Source: CAD feature listing. Evaluate the final solid. Frame: model axes, mm. A direction names the side the tool comes from. Coordinates: 2 decimals unless noted, no trailing zeros. Loops run counter-clockwise (first coordinate to the right, second up) from the corner with the lowest first, then second, coordinate; pieces in that order, holes last.
Item 1: Section query A-A, the plane y = 84.5. Return the cut outline in (x, z).
Item 2: Pull-direction query (X, two-part tool) for faces 3 (the flat face through (80, 59, 26)), 4 (the flat face through (78.5, 61, 26)), 5 (the flat face through (74, 121.5, 26)); classes: +X half, -X half, draft (parallel to the pull), parting line (faces both ways), or undercut.
Item 3: Section query B-B, the plane x = 7. Return the cut outline in (y, z), then the cut area to 3 significant figures.
Item 4: Reachability of faces 1 (the flat face through (-74, 121.5, 26)), 2 (the flat face through (1, 0, 20)) from +Z, -Z, +X, -X, +Y, -Y: full face, straight path, thin tool, end or side. Return the list, or none.
Item 5: Pin query (flat end, axial travel): pin 1 Ø1.2 at (y, z) = (-1, 45) entering from -X; pin 2 Ø1.2 at (y, z) = (-1, 45.5) entering from +X; pin 3 Ø1.6 at (y, z) = (120.5, 38.5) entering from +X. Return the tip coordinate at first contact, or that it passes through.
Item 6: Section query C-C, the plane z = 32.5. Return the cut outline in (x, y).
Item 7: Line query: probe 1 along X at (y, z) = (40, 35.5); probe 2 along Y at (x, z) = (-66, 12). Output: solid intervals per line, ascending.
```python
from build123d import *

# Parameters (mm, degrees)
F1_DEPTH = 52
F3_DEPTH = 123.001


with BuildPart() as f1:
    # F0 (on Top) → F1 (new body)
    with BuildSketch(Plane.XY):
        with BuildLine():
            Line((78, 0), (0, 0))
            Line((0, 0), (-78, 0))
            ThreePointArc((-78, 0), (-78.353553, 0.146447), (-78.5, 0.5))
            Line((-78.5, 0.5), (-78.5, 119.5))
            ThreePointArc((-78.5, 119.5), (-78.353553, 119.853553), (-78, 120))
            Line((-78, 120), (-70, 120))
            Line((-70, 120), (-70, 121.5))
            Line((-70, 121.5), (-78, 121.5))
            ThreePointArc((-78, 121.5), (-79.414214, 120.914214), (-80, 119.5))
            Line((-80, 119.5), (-80, 0.5))
            ThreePointArc((-80, 0.5), (-79.414214, -0.914214), (-78, -1.5))
            Line((-78, -1.5), (0, -1.5))
            Line((0, -1.5), (78, -1.5))
            ThreePointArc((78, -1.5), (79.414214, -0.914214), (80, 0.5))
            Line((80, 0.5), (80, 119.5))
            ThreePointArc((80, 119.5), (79.414214, 120.914214), (78, 121.5))
            Line((78, 121.5), (70, 121.5))
            Line((70, 121.5), (70, 120))
            Line((70, 120), (78, 120))
            ThreePointArc((78, 120), (78.353553, 119.853553), (78.5, 119.5))
            Line((78.5, 119.5), (78.5, 0.5))
            ThreePointArc((78.5, 0.5), (78.353553, 0.146447), (78, 0))
        make_face()
    extrude(amount=F1_DEPTH)

    # F2 (on face) → F3 (cut, through all)
    with BuildSketch(Plane.XZ.offset(1.5)):
        Polygon((0, 50), (-70, 50), (-70, 42), (0, 42), (70, 42), (70, 50), align=None)
    extrude(amount=-F3_DEPTH, mode=Mode.SUBTRACT)


solid = f1.part
```
Verdict:
1. outline: (-80, 0) - (-78.5, 0) - (-78.5, 52) - (-80, 52) - close; (78.5, 0) - (80, 0) - (80, 52) - (78.5, 52) - close
2. face 3: +X half
2. face 4: undercut
2. face 5: draft
3. outline: (-1.5, 0) - (0, 0) - (0, 42) - (-1.5, 42) - close; (-1.5, 50) - (0, 50) - (0, 52) - (-1.5, 52) - close
3. area: 66.0 mm2
4. face 1: +Z, -Z, +X, -X, +Y
4. face 2: +Z, -Z
5. pin 1: stops at x = -79.79
5. pin 2: stops at x = 79.79
5. pin 3: stops at x = 79.99
6. outline: (-80, 0.5) arc R2 ccw to (-78, -1.5) - (78, -1.5) arc R2 ccw to (80, 0.5) - (80, 119.5) arc R2 ccw to (78, 121.5) - (70, 121.5) - (70, 120) - (78, 120) arc R0.5 cw to (78.5, 119.5) - (78.5, 0.5) arc R0.5 cw to (78, 0) - (-78, 0) arc R0.5 cw to (-78.5, 0.5) - (-78.5, 119.5) arc R0.5 cw to (-78, 120) - (-70, 120) - (-70, 121.5) - (-78, 121.5) arc R2 ccw to (-80, 119.5) - close
7. probe 1: x = -80 to -78.5, 78.5 to 80
7. probe 2: y = -1.5 to 0
